Can you work these out from the model? Positions are in its coordinate system, mm. A direction names the side the tool comes from. Round coordinates to 2 decimals unless told otherwise and drop trailing zeros. Write each loop counter-clockwise with the first axis right and the second up, starting at its lowest first coordinate (ties: lowest second). Pieces come first, ordered by that corner, then holes. Notation, with made-up numbers: (80.5, 22) -> (133.5, 22) arc R25 ccw to (133.5, 57) -> close; hole circle Ø5 at (-2.75, 76). An arc over 180 degrees is marked (long way). Write item = value, one per line. Start each with the question number.
1) Thinking about a two-plate mould opening in X: for faces 1 (the face through (285.063, 440, -698)), 2 (the face through (379, 412.098, -698)), 3 (the face through (315, 461.098, -694)), which applies, +X half, -X half, draft (parallel to the pull), parting line (faces both ways), or undercut?
2) Imagine slicing it at B-B, the plane x = 396. Please give me the cut outline in (y, z), then the cut area to 3 significant figures.
3) For faces 4 (the face through (311, 467.098, -698)), 5 (the face through (470.461, 445, -694)), 6 (the face through (291.063, 438, -694)), 7 (the face through (476.461, 444, -698)), which set-ups out of +Z, -Z, +X, -X, +Y, -Y let a thin tool reach every point of the face, with its end or its side?
4) If I drill on line 1 (X direction, y = 429, z = -688); line 2 (Y direction, x = 465, z = -685.5); line 3 (Y direction, x = 319, z = -694.5), over which ranges is the centre line in solid material (lowest first)?
5) Imagine slicing it at D-D, the plane x = 438. Please give me the cut outline in (y, z).
6) I'm going to push flat-ended pins straight in: pin 1 (2 mm diameter, centred on y = 472.5, z = -707.5, fed in from -X); pin 2 (1.5 mm diameter, centred on x = 330, z = -709, fed in from +Y); pin 3 (5 mm diameter, centred on x = 393.5, y = 439.5, fed in from +Z); pin 4 (23.5 mm diameter, centred on x = 305.5, z = -683.5, fed in from -Y). Where does each tip first touch, or does it pass through?
7) Imagine slicing it at C-C, the plane y = 430.5. Please give me the cut outline in (x, z), then the cut area to 3 significant figures.
from build123d import *

# Parameters (mm, degrees)
BOSS_EXTRUDE1_DEPTH     = 4
BOSS_EXTRUDE2_DEPTH     = 50
CUT_EXTRUDE1_DEPTH      = 677.427541211
CUT_EXTRUDE1_DEPTH_BACK = 50
SKETCH3_W               = 18
SKETCH3_H               = 6
FILLET3_R               = 3


with BuildPart() as part:
    # Sketch1 → Boss-Extrude1 (new body)
    with BuildSketch(Plane.XY.offset(-724.191392871)):
        Polygon((476.461364297, 467.098298929), (476.461364297, 412.098298929), (285.063110998, 412.098298929), (285.063110998, 467.098298929), (337.030633325, 467.098298929), (337.030633325, 477.098298929), (476.461364297, 477.098298929), align=None)
    extrude(amount=BOSS_EXTRUDE1_DEPTH)

    # Sketch2 → Boss-Extrude2 (add)
    with BuildSketch(Plane.XY.offset(-720.191392871)):
        Polygon((285.063110998, 467.098298929), (285.063110998, 412.098298929), (476.461364297, 412.098298929), (476.461364297, 477.098298929), (337.030633325, 477.098298929), (337.030633325, 467.098298929), align=None)
        Polygon((291.063110998, 461.098298929), (343.030633325, 461.098298929), (343.030633325, 471.098298929), (470.461364297, 471.098298929), (470.461364297, 418.098298929), (291.063110998, 418.098298929), align=None, mode=Mode.SUBTRACT)
    extrude(amount=BOSS_EXTRUDE2_DEPTH)

    # Sketch3 → Cut-Extrude1 (cut, two sides: drawn at the far end of the back side and taken through both)
    with BuildSketch(Plane.XY.offset(-670.191392871).offset(-CUT_EXTRUDE1_DEPTH_BACK)):
        with Locations((300.063110998, 415.098298929)):
            Rectangle(SKETCH3_W, SKETCH3_H)
        with Locations((434.858034082, 415.098298929)):
            Rectangle(SKETCH3_W, SKETCH3_H)
    extrude(amount=CUT_EXTRUDE1_DEPTH + CUT_EXTRUDE1_DEPTH_BACK, mode=Mode.SUBTRACT)

    # Fillet3
    fillet3_edges = [part.edges().sort_by_distance(p)[0] for p in [
        (337.030633325, 477.098298929, -697.191392871),
        (476.461364297, 477.098298929, -697.191392871),
        (476.461364297, 412.098298929, -697.191392871),
        (285.063110998, 412.098298929, -697.191392871),
        (285.063110998, 467.098298929, -697.191392871),
        (337.030633325, 467.098298929, -697.191392871),
        (343.030633325, 461.098298929, -695.191392871),
        (406.745998811, 471.098298929, -720.191392871),
        (343.030633325, 466.098298929, -720.191392871),
        (317.046872162, 461.098298929, -720.191392871),
        (291.063110998, 436.598298929, -720.191392871),
        (470.461364297, 444.598298929, -720.191392871),
        (367.46057254, 418.098298929, -720.191392871),
        (457.159699189, 418.098298929, -720.191392871),
        (309.063110998, 418.098298929, -695.191392871),
        (309.063110998, 415.098298929, -720.191392871),
        (309.063110998, 412.098298929, -695.191392871),
        (291.063110998, 412.098298929, -695.191392871),
        (300.063110998, 412.098298929, -720.191392871),
        (425.858034082, 412.098298929, -695.191392871),
        (425.858034082, 415.098298929, -720.191392871),
        (425.858034082, 418.098298929, -695.191392871),
        (443.858034082, 412.098298929, -695.191392871),
        (443.858034082, 415.098298929, -720.191392871),
        (434.858034082, 412.098298929, -720.191392871),
    ]]
    fillet(fillet3_edges, radius=FILLET3_R - 0.0001)  # a hair under: the kernel refuses the full size


solid = part.part
Reported:
q1.face_1 = -X half
q1.face_2 = draft
q1.face_3 = undercut
q2.outline = (412.1, -724.19) -> (477.1, -724.19) -> (477.1, -670.19) -> (471.1, -670.19) -> (471.1, -717.19) arc R3 cw to (468.1, -720.19) -> (421.1, -720.19) arc R3 cw to (418.1, -717.19) -> (418.1, -670.19) -> (412.1, -670.19) -> close
q2.area = 864 mm²
q3.face_4 = +Z, -Z, -X, +Y
q3.face_5 = +Z
q3.face_6 = +Z, -Y
q3.face_7 = +Z, -Z, +X, +Y, -Y
q4.line_1 = 285.06 to 291.06, 470.46 to 476.46
q4.line_2 = 412.1 to 418.1, 471.1 to 477.1
q4.line_3 = 412.1 to 418.1, 461.1 to 467.1
q5.outline = (412.1, -724.19) -> (477.1, -724.19) -> (477.1, -670.19) -> (471.1, -670.19) -> (471.1, -717.19) arc R3 cw to (468.1, -720.19) -> (415.1, -720.19) arc R3 ccw to (412.1, -723.19) -> close
q6.pin_1 = 337.03
q6.pin_2 = 467.1
q6.pin_3 = -720.19
q6.pin_4 = 412.1
q7.outline = (285.06, -724.19) -> (476.46, -724.19) -> (476.46, -670.19) -> (470.46, -670.19) -> (470.46, -717.19) arc R3 cw to (467.46, -720.19) -> (294.06, -720.19) arc R3 cw to (291.06, -717.19) -> (291.06, -670.19) -> (285.06, -670.19) -> close
q7.area = 1,370 mm²
